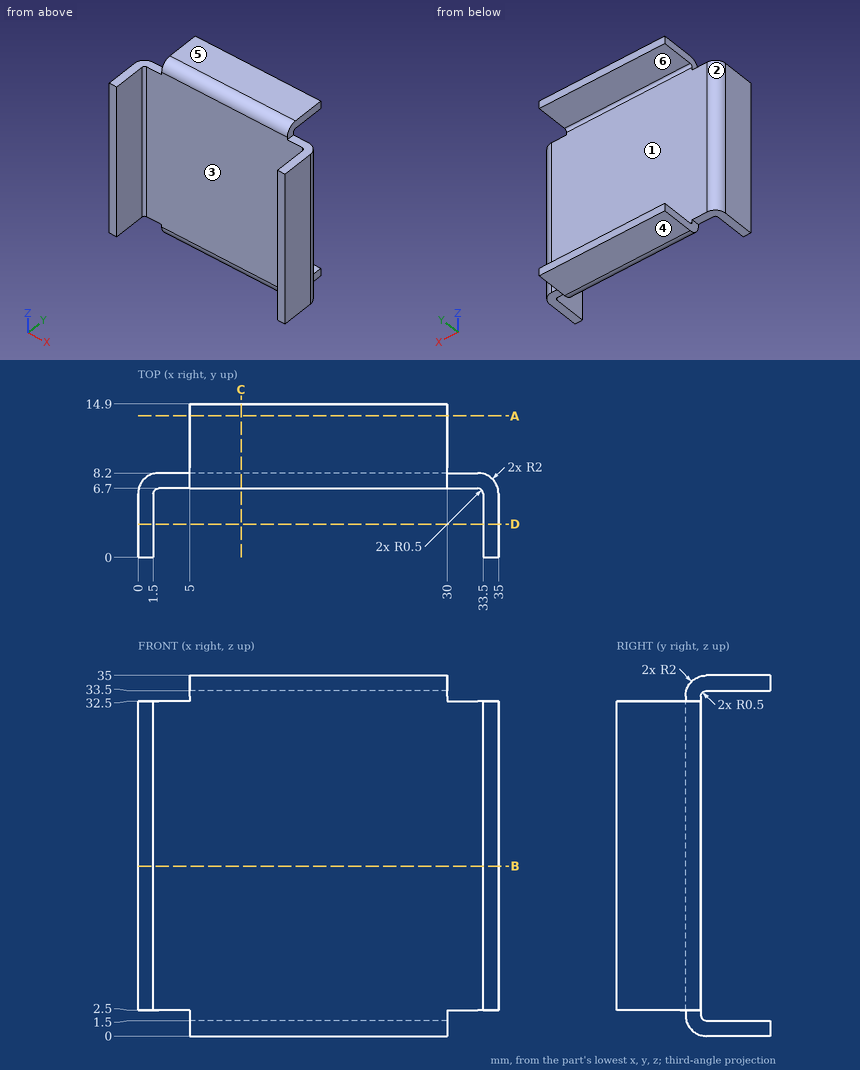
Study the drawing (mm; zero at the part's minimum x, y, z) and answer. A direction names the side the tool comes from. Coordinates: 2 decimals unless noted, no trailing zeros. Write each loop counter-clockwise with the first axis right and the second up, starting at its lowest first coordinate (ties: lowest second). Pieces come first, ordered by that corner, then holes.
Q1. A cutting plane is placed at A-A, the plane y = 13.75. Give the vertices of the cut face in (x, z), then the cut area to 3 significant figures.
Q2. Determine the mould class of the marked faces 4, 5 and 6 for opening direction Z: released by +Z, released by -Z, zero draft, split by the parting line, or undercut.
Q3. Which of the six approach directions +Z, -Z, +X, -X, +Y, -Y give full straight-line access (tool end or side, diameter ignored) to the marked faces 1, 2 and 3?
Q4. A cutting plane is placed at C-C, the plane x = 10. Give the vertices of the cut face in (y, z).
Q5. A cutting plane is placed at D-D, the plane y = 3.25. Give the vertices of the cut face in (x, z).
Q6. Each of these flat-tipped pins is pushed along its axis until it touches: pin 1 Ø4 at (x, z) = (23.5, 16.5) entering from -Y; pin 2 Ø4 at (x, y) = (6.5, 3.5) entering from -Z; pin 3 Ø1.2 at (y, z) = (11.5, 1.5) entering from +X; pin 4 Ø4 at (x, y) = (32, 5) entering from +Z. Where does it stop, or does it pass through?
Q7. A cutting plane is placed at B-B, the plane z = 16.5. Give the vertices of the cut face in (x, y).
Q8. Find the intervals of material crossed by line 1 (X direction, y = 2.5, z = 22); line 2 (Y direction, x = 4.5, z = 17.5), in increasing order.
Findings below:
1. outline: (5, 0) - (30, 0) - (30, 1.5) - (5, 1.5) - close; (5, 33.5) - (30, 33.5) - (30, 35) - (5, 35) - close
1. area: 75.0 mm2
2. face 4: released by -Z
2. face 5: released by +Z
2. face 6: undercut
3. face 1: +X, -X, +Y
3. face 2: +Z, -Z, -X, +Y
3. face 3: +Z, -Z, -Y
4. outline: (6.7, 2) arc R2 ccw to (8.7, 0) - (14.9, 0) - (14.9, 1.5) - (8.7, 1.5) arc R0.5 cw to (8.2, 2) - (8.2, 33) arc R0.5 cw to (8.7, 33.5) - (14.9, 33.5) - (14.9, 35) - (8.7, 35) arc R2 ccw to (6.7, 33) - close
5. outline: (0, 2.5) - (1.5, 2.5) - (1.5, 32.5) - (0, 32.5) - close; (33.5, 2.5) - (35, 2.5) - (35, 32.5) - (33.5, 32.5) - close
6. pin 1: stops at y = 6.7
6. pin 2: passes through
6. pin 3: stops at x = 30
6. pin 4: stops at z = 32.5
7. outline: (0, 0) - (1.5, 0) - (1.5, 6.2) arc R0.5 cw to (2, 6.7) - (33, 6.7) arc R0.5 cw to (33.5, 6.2) - (33.5, 0) - (35, 0) - (35, 6.2) arc R2 ccw to (33, 8.2) - (2, 8.2) arc R2 ccw to (0, 6.2) - close
8. line 1: x = 0 to 1.5, 33.5 to 35
8. line 2: y = 6.7 to 8.2
